The model under review builds one solid part; all positions refer to its coordinate system, in mm. A direction names the side the tool comes from. Round coordinates to 2 decimals unless told otherwise and drop trailing zeros. Loops run counter-clockwise (first coordinate to the right, second up) from the corner with the lowest first, then second, coordinate; pieces in that order, holes last. Notation, with made-up numbers: (10.25, -25) -> (29.25, -25) arc R16 cw to (29.25, -12) -> close; hole circle Ø1 at (80.5, -16.5). An arc over 180 degrees is marked (long way). Write each question's results on one line, items separated by ' | '. Start each with the question number.
Item 1: For L1, parallel to Y at x = 1.5, z = -5.25; L2, parallel to Y at x = 10.25, z = 12.75; L3, parallel to Y at x = 6.5, z = 9.5, list the stretches that pass through material, from the lowest coordinate up. Write a range as from..to.
Item 2: We need section C-C (y = 1.5). Give the boundary of the cut face in (x, z).
Item 3: Clearance check with flat-ended pins moving along their axes: pin 1 Ø1 at (x, z) = (3, -8.5) entering from -Y; pin 2 Ø1.5 at (y, z) = (-7.5, -6.5) entering from +X; pin 3 Ø3.5 at (x, y) = (7.5, 1) entering from +Z; pin 4 Ø0.6 at (y, z) = (0, -8.5) entering from -X. State where each tip first meets the part, or that it passes through.
Item 4: Mouldability with a two-part tool opening along Y and no side actions: class faces 1 (the flat face through (5, -5.323, -2)), 2 (the cylindrical face through (5.58, 7.38, 5.34)), 3 (the cylindrical face through (5.42, 2.88, -7.46)), 4 (the cylindrical face through (5, -4, 7)) as pulls with the +Y half, pulls with the -Y half, needs draft (parallel to the pull), parting line crosses it, or undercut.
Item 5: We need section B-B (z = 5.75). Give the boundary of the cut face in (x, y), and give its area (3 significant figures).
Item 6: We need section A-A (z = 1.5). Give the boundary of the cut face in (x, y), and give its area (3 significant figures).
Item 7: We need section D-D (y = -10). Give the boundary of the cut face in (x, z).
Item 8: Tool access review of faces 5 (the flat face through (5.42, -7.84, 8.57)), 6 (the flat face through (5, 5.177, -2)), 7 (the flat face through (4, -1.073, -9)): name each direction out of +Z, -Z, +X, -X, +Y, -Y from which nothing blocks a thin tool from reaching the whole face with its end or side.
from build123d import *

# Parameters (mm, degrees)
BOSS_EXTRUDE1_DEPTH = 11
SKETCH2_W           = 6.5
SKETCH2_H           = 2
CUT_EXTRUDE1_DEPTH  = 11
SKETCH3_W           = 11
SKETCH3_H           = 2
BOSS_EXTRUDE2_DEPTH = 2.5
SKETCH4_W           = 7.103618525
SKETCH4_H           = 2.480120743
CUT_EXTRUDE2_DEPTH  = 32.5
SKETCH5_W           = 11
SKETCH5_H           = 2
BOSS_EXTRUDE3_DEPTH = 5
SKETCH6_W           = 11
SKETCH6_H           = 1
BOSS_EXTRUDE4_DEPTH = 1.5
CHAMFER1_SIZE       = 0.5
SKETCH7_W           = 11
SKETCH7_H           = 2
BOSS_EXTRUDE5_DEPTH = 6
SKETCH8_W           = 9.245207015
SKETCH8_H           = 4.24468792
CUT_EXTRUDE3_DEPTH  = 26
SKETCH9_W           = 11
SKETCH9_H           = 2
BOSS_EXTRUDE6_DEPTH = 7
SKETCH10_W          = 11
SKETCH10_H          = 1
BOSS_EXTRUDE7_DEPTH = 1
CHAMFER2_SIZE       = 0.5
FILLET1_R           = 1
CHAMFER3_SIZE       = 0.5
CHAMFER4_SIZE       = 1
SKETCH11_W          = 2.25
SKETCH11_H          = 2
CUT_EXTRUDE4_DEPTH  = 10
FILLET2_R           = 0.6
CHAMFER5_SIZE       = 3
CHAMFER6_SIZE       = 4
CHAMFER7_SIZE       = 0.5


with BuildPart() as part:
    # Sketch1 → Boss-Extrude1 (new body)
    with BuildSketch(Plane(origin=(0, 0, 0), x_dir=(0, 0, -1), z_dir=(1, 0, 0))):
        with BuildLine():
            Line((-12.25399361, 3.177316294), (-12.25399361, 5.177316294))
            Line((-12.25399361, 5.177316294), (8.74600639, 5.177316294))
            ThreePointArc((8.74600639, 5.177316294), (9.453113171, 4.884423075), (9.74600639, 4.177316294))
            Line((9.74600639, 4.177316294), (9.74600639, -4.322683706))
            ThreePointArc((9.74600639, -4.322683706), (9.453113171, -5.029790487), (8.74600639, -5.322683706))
            Line((8.74600639, -5.322683706), (-12.25399361, -5.322683706))
            Line((-12.25399361, -5.322683706), (-12.25399361, -3.322683706))
            Line((-12.25399361, -3.322683706), (6.74600639, -3.322683706))
            ThreePointArc((6.74600639, -3.322683706), (7.453113171, -3.029790487), (7.74600639, -2.322683706))
            Line((7.74600639, -2.322683706), (7.74600639, 2.177316294))
            ThreePointArc((7.74600639, 2.177316294), (7.453113171, 2.884423075), (6.74600639, 3.177316294))
            Line((6.74600639, 3.177316294), (-12.25399361, 3.177316294))
        make_face()
    extrude(amount=BOSS_EXTRUDE1_DEPTH)

    # Sketch2 → Cut-Extrude1 (cut)
    with BuildSketch(Plane.XY.offset(-7.74600639)):
        with Locations((5.5, -0.072683706)):
            Rectangle(SKETCH2_W, SKETCH2_H)
    extrude(amount=-CUT_EXTRUDE1_DEPTH, mode=Mode.SUBTRACT)

    # Sketch3 → Boss-Extrude2 (add)
    with BuildSketch(Plane(origin=(0, 5.177316294, 0), x_dir=(1, 0, 0), z_dir=(0, 1, 0))):
        with Locations((5.5, -6.05399361)):
            Rectangle(SKETCH3_W, SKETCH3_H)
    extrude(amount=BOSS_EXTRUDE2_DEPTH)

    # Sketch4 → Cut-Extrude2 (cut)
    with BuildSketch(Plane.ZY):
        with Locations((10.605802872, 3.937255923)):
            Rectangle(SKETCH4_W, SKETCH4_H)
    extrude(amount=-CUT_EXTRUDE2_DEPTH, mode=Mode.SUBTRACT)

    # Sketch5 → Boss-Extrude3 (add)
    with BuildSketch(Plane.XY.offset(7.05399361)):
        with Locations((5.5, 6.677316294)):
            Rectangle(SKETCH5_W, SKETCH5_H)
    extrude(amount=BOSS_EXTRUDE3_DEPTH)

    # Sketch6 → Boss-Extrude4 (add)
    with BuildSketch(Plane.XZ.offset(-5.677316294)):
        with Locations((5.5, 11.55399361)):
            Rectangle(SKETCH6_W, SKETCH6_H)
    extrude(amount=BOSS_EXTRUDE4_DEPTH)

    # Chamfer1
    chamfer1_edges = [part.edges().sort_by_distance(p)[0] for p in [
        (5.5, 4.177316294, 12.05399361),
    ]]
    chamfer(chamfer1_edges, length=CHAMFER1_SIZE)

    # Sketch7 → Boss-Extrude5 (add)
    with BuildSketch(Plane.XZ.offset(5.322683706)):
        with Locations((5.5, 6.05399361)):
            Rectangle(SKETCH7_W, SKETCH7_H)
    extrude(amount=BOSS_EXTRUDE5_DEPTH)

    # Sketch8 → Cut-Extrude3 (cut)
    with BuildSketch(Plane(origin=(11, 0, 0), x_dir=(0, 0, -1), z_dir=(1, 0, 0))):
        with Locations((-11.676597118, -3.200339746)):
            Rectangle(SKETCH8_W, SKETCH8_H)
    extrude(amount=-CUT_EXTRUDE3_DEPTH, mode=Mode.SUBTRACT)

    # Sketch9 → Boss-Extrude6 (add)
    with BuildSketch(Plane.XY.offset(7.05399361)):
        with Locations((5.5, -10.322683706)):
            Rectangle(SKETCH9_W, SKETCH9_H)
    extrude(amount=BOSS_EXTRUDE6_DEPTH)

    # Sketch10 → Boss-Extrude7 (add)
    with BuildSketch(Plane(origin=(0, -9.322683706, 0), x_dir=(1, 0, 0), z_dir=(0, 1, 0))):
        with Locations((5.5, -13.55399361)):
            Rectangle(SKETCH10_W, SKETCH10_H)
    extrude(amount=BOSS_EXTRUDE7_DEPTH)

    # Chamfer2
    chamfer2_edges = [part.edges().sort_by_distance(p)[0] for p in [
        (5.5, -8.322683706, 14.05399361),
    ]]
    chamfer(chamfer2_edges, length=CHAMFER2_SIZE)

    # Fillet1
    fillet1_edges = [part.edges().sort_by_distance(p)[0] for p in [
        (5.5, -3.322683706, 7.05399361),
        (5.5, 7.677316294, 5.05399361),
        (5.5, 3.177316294, 7.05399361),
    ]]
    fillet(fillet1_edges, radius=FILLET1_R)

    # Chamfer3
    chamfer3_edges = [part.edges().sort_by_distance(p)[0] for p in [
        (5.5, -11.322683706, 14.05399361),
        (5.5, 7.677316294, 12.05399361),
    ]]
    chamfer(chamfer3_edges, length=CHAMFER3_SIZE)

    # Chamfer4
    chamfer4_edges = [part.edges().sort_by_distance(p)[0] for p in [
        (5.5, -5.322683706, 5.05399361),
        (5.5, 5.177316294, 5.05399361),
    ]]
    chamfer(chamfer4_edges, length=CHAMFER4_SIZE)

    # Sketch11 → Cut-Extrude4 (cut)
    with BuildSketch(Plane(origin=(0, 0, -9.74600639), x_dir=(-1, 0, 0), z_dir=(0, 0, -1))):
        with Locations((-1.125, -0.072683706)):
            Rectangle(SKETCH11_W, SKETCH11_H)
    extrude(amount=-CUT_EXTRUDE4_DEPTH, mode=Mode.SUBTRACT)

    # Fillet2
    fillet2_edges = [part.edges().sort_by_distance(p)[0] for p in [
        (8.75, 0.927316294, -8.74600639),
        (8.75, -1.072683706, -8.74600639),
    ]]
    fillet(fillet2_edges, radius=FILLET2_R)

    # Chamfer5
    chamfer5_edges = [part.edges().sort_by_distance(p)[0] for p in [
        (5.5, -9.322683706, 7.05399361),
    ]]
    chamfer(chamfer5_edges, length=CHAMFER5_SIZE)

    # Chamfer6
    chamfer6_edges = [part.edges().sort_by_distance(p)[0] for p in [
        (5.5, -11.322683706, 5.05399361),
    ]]
    chamfer(chamfer6_edges, length=CHAMFER6_SIZE)

    # Chamfer7
    chamfer7_edges = [part.edges().sort_by_distance(p)[0] for p in [
        (5.5, 5.677316294, 7.05399361),
    ]]
    chamfer(chamfer7_edges, length=CHAMFER7_SIZE)


solid = part.part
Here are the results:
1) L1: y = -5.32..-3.32, 3.18..5.18 | L2: y = -11.32..-9.32 | L3: y = -11.32..-8.77, 5.68..7.68
2) outline: (0, -9.75) -> (11, -9.75) -> (11, -7.75) -> (0, -7.75) -> close
3) pin 1: stops at y = -5.32 | pin 2: passes through | pin 3: stops at z = -7.57 | pin 4: stops at x = 8.75
4) face 1: pulls with the -Y half | face 2: pulls with the +Y half | face 3: undercut | face 4: undercut
5) outline: (0, -8.02) -> (11, -8.02) -> (11, -3.32) -> (0, -3.32) -> close; (0, 3.18) -> (11, 3.18) -> (11, 7.63) -> (0, 7.63) -> close | area: 101 mm2
6) outline: (0, -5.32) -> (11, -5.32) -> (11, -3.32) -> (0, -3.32) -> close; (0, 3.18) -> (11, 3.18) -> (11, 5.18) -> (0, 5.18) -> close | area: 44.0 mm2
7) outline: (0, 7.73) -> (11, 7.73) -> (11, 14.05) -> (0, 14.05) -> close
8) face 5: +X, -X | face 6: -Z, +X, -X, +Y | face 7: +Z, -Z, -X
